```python
from build123d import *

# Parameters (mm, degrees)
F0_W           = 157
F0_H           = 157
F1_DEPTH       = 10
F2_W           = 151
F2_H           = 151
F3_DEPTH       = 7
F5_D           = 9
F5_CSINK_D     = 10
F5_CSINK_ANGLE = 90
F6_R           = 10
F7_R           = 10
F8_R           = 10


# Not quite as in the source:
# - a feature names something its author has since deleted; it is built from what else it names


with BuildPart() as f1:
    # F0 (on Top) → F1 (new body)
    with BuildSketch(Plane.XY):
        Rectangle(F0_W, F0_H)
    extrude(amount=F1_DEPTH)

    # F2 (on Top) → F3 (cut)
    with BuildSketch(Plane.XY):
        Rectangle(F2_W, F2_H)
    extrude(amount=F3_DEPTH, mode=Mode.SUBTRACT)

    # F5 (through all)
    with Locations(Plane(origin=(0, 0, 0), x_dir=(1, 0, 0), z_dir=(0, 0, -1))):
        with Locations((0, 0), (0, -19.7167731822), (0, -37.2098498046), (0, -51.4415055513), (0, -65.3766617179), (17.9378120229, 0), (41.9537350535, 0), (68.3415979147, 0), (-18.8272930682, 0), (-42.8432114422, 0), (-65.6731575727, 0), (0, 17.6413226873), (0, 35.1343974471), (0, 51.1450096965), (41.9537350535, -36.9133576751), (68.3415979147, -65.3766617179), (68.3415979147, -52.3309856653), (68.3415979147, -36.9133576751), (68.3415979147, -20.0132653117), (18.234308809, -19.7167731822), (17.9378120229, -36.9133576751), (41.9537350535, -52.3309856653), (41.9537350535, -65.3766617179), (17.9378120229, -52.3309856653), (-19.7167731822, -65.3766617179), (-65.9696534276, -65.3766617179), (17.9378120229, -65.3766617179), (41.9537350535, -20.0132653117), (-19.4202791899, -52.3309856653), (-19.4202791899, -36.9133576751), (-19.1237870604, -19.7167731822), (-65.9696534276, -19.7167731822), (-65.9696534276, -36.9133576751), (-65.9696534276, -51.7380014062), (-44.3256758153, -51.7380014062), (-44.3256758153, -36.9133576751), (-44.3256758153, -19.123788923), (-44.3256758153, -65.3766617179), (-65.6731575727, 68.638086319), (-65.6731575727, 51.1450096965), (-65.6731575727, 35.1343974471), (-65.6731575727, 17.6413226873), (-42.8432114422, 17.6413226873), (-42.8432114422, 35.1343974471), (-18.8272930682, 35.1343974471), (-18.8272930682, 17.6413226873), (-42.8432114422, 68.638086319), (-18.8272930682, 68.638086319), (-18.8272930682, 51.1450096965), (18.8272949308, 51.1450096965), (17.9378120229, 35.1343974471), (17.9378120229, 17.6413226873), (41.9537350535, 17.6413226873), (68.3415979147, 17.6413226873), (68.3415979147, 35.1343974471), (41.9537350535, 35.1343974471), (43.4361994267, 51.1450096965), (18.8272949308, 68.638086319), (0, 68.638086319), (43.4361994267, 68.638086319), (67.4521178007, 68.638086319), (67.4521178007, 51.1450096965), (-42.8432114422, 51.1450096965)):
            CounterSinkHole(F5_D / 2, F5_CSINK_D / 2, counter_sink_angle=F5_CSINK_ANGLE)

    # F6
    f6_edges = [f1.edges().sort_by_distance(p)[0] for p in [
        (78.5, 78.5, 5),
        (-78.5, 78.5, 5),
        (78.5, -78.5, 5),
    ]]
    fillet(f6_edges, radius=F6_R)

    # F7
    f7_edges = [f1.edges().sort_by_distance(p)[0] for p in [
        (-78.5, -78.5, 5),
    ]]
    fillet(f7_edges, radius=F7_R)

    # F8
    f8_edges = [f1.edges().sort_by_distance(p)[0] for p in [
        (75.5, -75.5, 3.5),
        (-75.5, -75.5, 3.5),
        (-75.5, 75.5, 3.5),
        (75.5, 75.5, 3.5),
    ]]
    fillet(f8_edges, radius=F8_R)


solid = f1.part
```
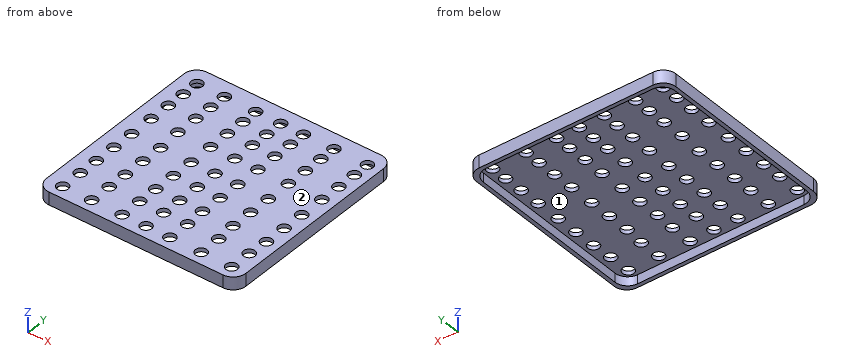
Can you work these out from the model? Positions are in its coordinate system, mm. Face numbers are marked on the shaded views. Round coordinates to 2 decimals unless told otherwise and drop trailing zeros. Order: outer loops, then holes, each group sorted by start corner. A loop starts at its lowest first (then second) coordinate and runs counter-clockwise, first axis right, second up. Notation, with made-up numbers: (-39.5, 79.5) -> (13.5, 79.5) arc R13 cw to (13.5, 90.5) -> close; hole circle Ø10 at (3, 48). An arc over 180 degrees is marked (long way). Return JSON: item names as keys, results as strings. Group by question number.
1. We'd pull the mould along X, two halves only. Please class the marked faces 1 and 2: released by +X, released by -X, zero draft, split by the parting line, or undercut.
2. If we section it at C-C, the plane z = 5.25: Write out the boundary of the cut face in (x, y), then the cut area to 3 significant figures.
3. If we section it at A-A, the plane y = 30.5: Write out the boundary of the cut face in (x, z), then the cut area to 3 significant figures.
4. If we section it at B-B, the plane x = 0: Count the separate pieces of the cut face and the enclosed holes in it, then the cut area to 3 significant figures.
5. I need wall thicknesses on line 1 (X direction, y = -49, z = 5.25); line 2 (Z direction, x = -14.5, y = 13). Which ranges of each line are inside material? Lowest first, please. Write a range as [from, to].
6. Will this pin go through, and if not, where does the flat tip stop? pin 1 (14.5 mm diameter, centred on x = -18.83, y = -17.64, fed in from -Z).
Output values:
{
 "1": {"face 1": "undercut", "face 2": "zero draft"},
 "2": {"outline": "(-78.5, -68.5) arc R10 ccw to (-68.5, -78.5) -> (68.5, -78.5) arc R10 ccw to (78.5, -68.5) -> (78.5, 68.5) arc R10 ccw to (68.5, 78.5) -> (-68.5, 78.5) arc R10 ccw to (-78.5, 68.5) -> close; hole (-75.5, -65.5) arc R10 ccw to (-65.5, -75.5) -> (65.5, -75.5) arc R10 ccw to (75.5, -65.5) -> (75.5, 65.5) arc R10 ccw to (65.5, 75.5) -> (-65.5, 75.5) arc R10 ccw to (-75.5, 65.5) -> close", "area": "1,850 mm²"},
 "3": {"outline": "(-78.5, 0) -> (-75.5, 0) -> (-75.5, 7) -> (75.5, 7) -> (75.5, 0) -> (78.5, 0) -> (78.5, 10) -> (-78.5, 10) -> close", "area": "513 mm²"},
 "4": {"separate pieces": "10", "enclosed holes": "0", "area": "270 mm²"},
 "5": {"line 1": "[-78.5, -75.5], [75.5, 78.5]", "line 2": "[7, 10]"},
 "6": {"pin 1": "z = 7"}
}
